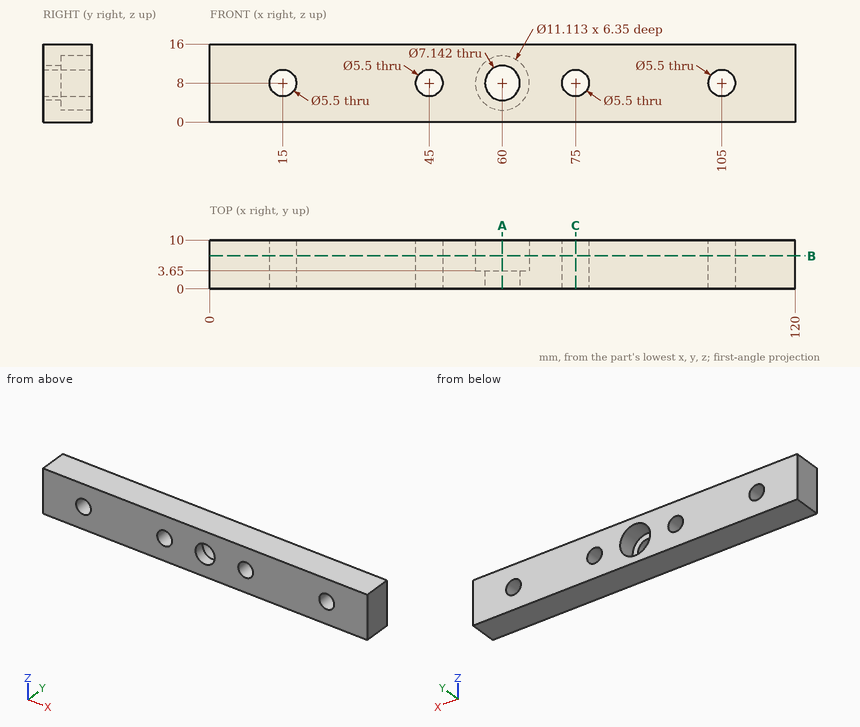
Drawing for the job (mm, zero at the part's lowest x, y, z). Round coordinates to 2 decimals unless told otherwise and drop trailing zeros. Loops run counter-clockwise (first coordinate to the right, second up) from the corner with the lowest first, then second, coordinate; pieces in that order, holes last. Notation, with made-up numbers: (23.25, 64) -> (77.25, 64) arc R24 ccw to (77.25, 102) -> close; hole circle Ø5 at (9.5, 80). An arc over 180 degrees is marked (long way). Answer as CSV lines item,"result". Start each with the question number.
1) Slice it at B-B (y = 6.75). List the corners of the cut face in (x, z), plus the area to 3 significant figures.
2) Probe line 1 along X through (y, z) = (7, 8); line 2 along X through (y, z) = (2, 8); line 3 along Z through (x, y) = (45, 4.75). List the from-to ranges inside material, lowest first.
3) Slice it at C-C (x = 75). List the corners of the cut face in (y, z), plus the area to 3 significant figures.
4) Pin check, flat tips, straight feed: P1, Ø8, axis at x = 60, z = 8, coming from the +Y side; P2, Ø3.5, axis at x = 105, z = 8, coming from the +Y side. Stop position of each tip, or through.
5) Slice it at A-A (x = 60). List the corners of the cut face in (y, z), plus the area to 3 significant figures.
Filled in:
1,outline,"(0, 0) -> (120, 0) -> (120, 16) -> (0, 16) -> close; hole circle Ø5.5 at (15, 8); hole circle Ø5.5 at (45, 8); hole circle Ø11.11 at (60, 8); hole circle Ø5.5 at (75, 8); hole circle Ø5.5 at (105, 8)"
1,area,"1,730 mm2"
2,line 1,"x = 0 to 12.25, 17.75 to 42.25, 47.75 to 54.44, 65.56 to 72.25, 77.75 to 102.25, 107.75 to 120"
2,line 2,"x = 0 to 12.25, 17.75 to 42.25, 47.75 to 56.43, 63.57 to 72.25, 77.75 to 102.25, 107.75 to 120"
2,line 3,"z = 0 to 5.25, 10.75 to 16"
3,outline,"(0, 0) -> (10, 0) -> (10, 5.25) -> (0, 5.25) -> close; (0, 10.75) -> (10, 10.75) -> (10, 16) -> (0, 16) -> close"
3,area,"105 mm2"
4,P1,"stops at y = 3.65"
4,P2,"passes through"
5,outline,"(0, 0) -> (10, 0) -> (10, 2.44) -> (3.65, 2.44) -> (3.65, 4.43) -> (0, 4.43) -> close; (0, 11.57) -> (3.65, 11.57) -> (3.65, 13.56) -> (10, 13.56) -> (10, 16) -> (0, 16) -> close"
5,area,"63.4 mm2"
